Geometry: see drawing. Coordinates: mm, zero at the bounding-box minimum. A direction names the side the tool comes from. Round coordinates to 2 decimals unless told otherwise and drop trailing zeros. Order: outer loops, then holes, each group sorted by start corner. A loop starts at its lowest first (then second) coordinate and runs counter-clockwise, first axis right, second up. Notation, with made-up numbers: (-17, 24) -> (33, 24) arc R15 cw to (33, 40) -> close; hole circle Ø4 at (9.25, 35.25). An arc over 180 degrees is marked (long way). Answer as CSV lines item,"result". Start each with the question number.
(1) Line query: line 1 along Z through (x, y) = (8.25, 7.5); line 2 along Y through (x, z) = (5, 31.5); line 3 along Y through (x, z) = (7, 34). Output: solid intervals per line, ascending. Write a range as from..to.
(2) Contact query for flat-ended pins moving along their axis: P1, Ø4.5, axis at y = 6.5, z = 23.5, coming from the -X side; P2, Ø4, axis at x = 2, z = 28.5, coming from the +Y side; P3, Ø1, axis at x = 6.5, y = 24, coming from the -Z side. Output: stop coordinate, or through.
(3) Section query B-B (x = 7.25). Output: boundary loops of the cut face in (y, z), plus the area to 3 significant figures.
(4) Set-up query: the marked faces 1 and 2. Return all of +Z, -Z, +X, -X, +Y, -Y with unobstructed straight access to the full face (end or side cutting, diameter ignored); none if empty.
(5) Section query A-A (z = 31.4). Output: boundary loops of the cut face in (x, y), plus the area to 3 significant figures.
(6) Section query C-C (z = 38). Output: boundary loops of the cut face in (x, y).
(7) Section query D-D (y = 7.5). Output: boundary loops of the cut face in (x, z).
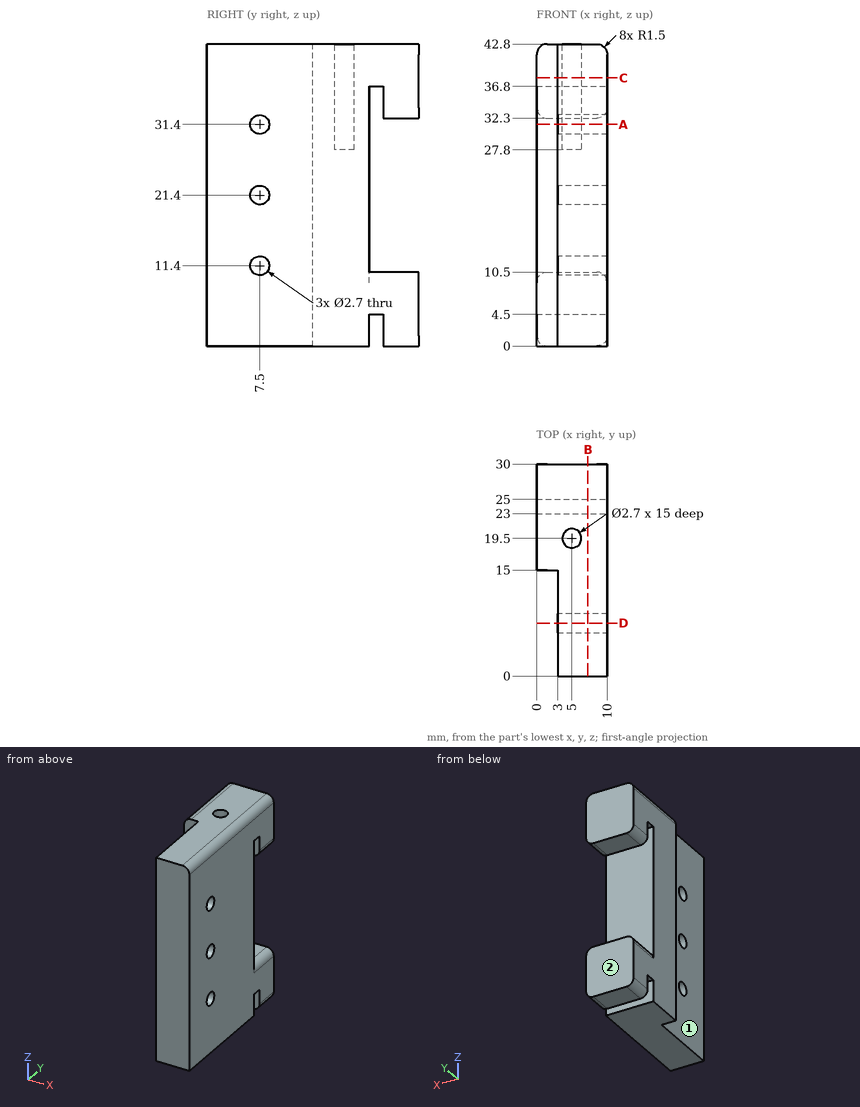
Answer block:
1,line 1,"0..10.05, 12.75..20.05, 22.75..30.05, 32.75..42.8"
1,line 2,"0..6.15, 8.85..18.15, 20.85..23"
1,line 3,"0..23, 25..30"
2,P1,"x = 3"
2,P2,"y = 23"
2,P3,"z = 4.5"
3,outline,"(0, 0) -> (23, 0) -> (23, 4.5) -> (25, 4.5) -> (25, 0) -> (30, 0) -> (30, 10.5) -> (23, 10.5) -> (23, 36.8) -> (25, 36.8) -> (25, 32.3) -> (30, 32.3) -> (30, 42.8) -> (0, 42.8) -> close; hole circle Ø2.7 at (7.5, 11.4); hole circle Ø2.7 at (7.5, 21.4); hole circle Ø2.7 at (7.5, 31.4)"
3,area,"1,100 mm2"
4,face 1,"+Z, -Z, -X, -Y"
4,face 2,"+Z, -Z, +X, -X, +Y"
5,outline,"(0, 15) -> (3, 15) -> (3, 8.85) -> (10, 8.85) -> (10, 23) -> (0, 23) -> close; (3, 0) -> (10, 0) -> (10, 6.15) -> (3, 6.15) -> close; hole circle Ø2.7 at (5, 19.5)"
5,area,"160 mm2"
6,outline,"(0, 15) -> (3, 15) -> (3, 0) -> (10, 0) -> (10, 30) -> (0, 30) -> close; hole circle Ø2.7 at (5, 19.5)"
7,outline,"(3, 0) -> (10, 0) -> (10, 10.05) -> (3, 10.05) -> close; (3, 12.75) -> (10, 12.75) -> (10, 20.05) -> (3, 20.05) -> close; (3, 22.75) -> (10, 22.75) -> (10, 30.05) -> (3, 30.05) -> close; (3, 32.75) -> (10, 32.75) -> (10, 41.3) arc R1.5 ccw to (8.5, 42.8) -> (3, 42.8) -> close"
